Check sheet for the modelled part. Datum: model origin and axes. Units: mm. A direction names the side the tool comes from. Round coordinates to 2 decimals unless told otherwise and drop trailing zeros. Write each loop counter-clockwise with the first axis right and the second up, starting at its lowest first coordinate (ties: lowest second). Pieces come first, ordered by that corner, then holes.
Item 1: Set-up check for faces 5 (the flat face through (2, 16, 15)), 6 (the flat face through (3, 25, 7)): record each of +Z, -Z, +X, -X, +Y, -Y from which the full face is reachable in a straight line by a thin tool's end or side.
Item 2: Depth check by flat-ended pin: pin 1 (2 mm diameter, centred on x = 1, y = 120, fed in from -Z); pin 2 (12 mm diameter, centred on y = -17, z = -0.5, fed in from +X); pin 3 (5 mm diameter, centred on x = 63, z = -11.5, fed in from +Y); pin 4 (1 mm diameter, centred on y = 56.5, z = -5, fed in from -X). Enter the tip coordinate at first touch or a pass-through.
Item 3: Section check B-B, the plane y = -55. Record the cut outline in (x, z).
Item 4: Material ranges on line 1 along Z through (x, y) = (30.5, -84.3); line 2 along Y through (x, z) = (1.6, 0); line 3 along Y through (x, z) = (95, -4), recorded low to high.
Item 5: Section check A-A, the plane x = 67.5. Record the cut outline in (y, z), plus the area to 3 significant figures.
Item 6: Section check C-C, the plane x = 85. Record the cut outline in (y, z).
Item 7: Section check D-D, the plane y = 47.5. Record the cut outline in (x, z).
Item 8: Release check for a two-part mould opening along Y. For faces 1 (the cylindrical face through (1.52, 131.99, 12.15)), 2 (the cylindrical face through (1.48, 67.07, -0.65)), 3 (the flat face through (51, -85, 10)), 4 (the flat face through (0, 23, 7)) record: pulls with the +Y half, pulls with the -Y half, needs draft (parallel to the pull), parting line crosses it, or undercut.
from build123d import *

# Parameters (mm, degrees)
SKETCH_1_W          = 30
SKETCH_1_H          = 170
EXTRUDE_1_DEPTH     = 3
SKETCH_2_W          = 30
SKETCH_2_H          = 3
EXTRUDE_2_DEPTH     = 100
SKETCH_4_R          = 1.6
SKETCH_4_R_2        = 3
CUT_EXTRUDE_1_DEPTH = 104
SKETCH_5_W          = 3
SKETCH_5_H          = 30
EXTRUDE_3_DEPTH     = 50
SKETCH_6_R          = 10.5
SKETCH_6_W          = 2
SKETCH_6_H          = 2.5
CUT_EXTRUDE_2_DEPTH = 104
FILLET_1_R          = 10
SKETCH_7_R          = 1.6
SKETCH_7_W          = 60
SKETCH_7_H          = 15
CUT_EXTRUDE_3_DEPTH = 4
FILLET_2_R          = 5
SKETCH_8_R          = 5
SKETCH_8_W          = 10
SKETCH_8_H          = 60
CUT_EXTRUDE_4_DEPTH = 104


with BuildPart() as part:
    # 草图1 → 凸台-拉伸1 (new body)
    with BuildSketch(Plane(origin=(0, 0, 0), x_dir=(0, 0, -1), z_dir=(1, 0, 0))):
        Rectangle(SKETCH_1_W, SKETCH_1_H)
    extrude(amount=EXTRUDE_1_DEPTH)

    # 草图2 → 凸台-拉伸2 (add)
    with BuildSketch(Plane(origin=(3, 0, 0), x_dir=(0, 0, -1), z_dir=(1, 0, 0))):
        with Locations((0, -83.5)):
            Rectangle(SKETCH_2_W, SKETCH_2_H)
    extrude(amount=EXTRUDE_2_DEPTH)

    # 草图4 → 切除-拉伸1 (cut, through all)
    with BuildSketch(Plane.ZY):
        with Locations((-4.949747468, 74.949747468)):
            Circle(SKETCH_4_R)
        with Locations((4.949747468, 74.949747468)):
            Circle(SKETCH_4_R)
        with Locations((4.949747468, 65.050252532)):
            Circle(SKETCH_4_R)
        with Locations((-4.949747468, 65.050252532)):
            Circle(SKETCH_4_R)
        with Locations((0, 70)):
            Circle(SKETCH_4_R_2)
    extrude(amount=-CUT_EXTRUDE_1_DEPTH, mode=Mode.SUBTRACT)

    # 草图5 → 凸台-拉伸3 (add)
    with BuildSketch(Plane(origin=(0, 85, 0), x_dir=(1, 0, 0), z_dir=(0, 1, 0))):
        with Locations((1.5, 0)):
            Rectangle(SKETCH_5_W, SKETCH_5_H)
    extrude(amount=EXTRUDE_3_DEPTH)

    # 草图6 → 切除-拉伸2 (cut, through all)
    with BuildSketch(Plane.ZY):
        with Locations((0, 120)):
            Circle(SKETCH_6_R)
        with Locations((-15, 120)):
            Rectangle(SKETCH_6_W, SKETCH_6_H)
        with Locations((15, 120)):
            Rectangle(SKETCH_6_W, SKETCH_6_H)
    extrude(amount=-CUT_EXTRUDE_2_DEPTH, mode=Mode.SUBTRACT)

    # 圆角1
    fillet_1_edges = [part.edges().sort_by_distance(p)[0] for p in [
        (1.5, 135, 15),
        (1.5, 135, -15),
    ]]
    fillet(fillet_1_edges, radius=FILLET_1_R)

    # 草图7 → 切除-拉伸3 (cut, through all)
    with BuildSketch(Plane(origin=(0, -82, 0), x_dir=(1, 0, 0), z_dir=(0, 1, 0))):
        with Locations((90.5, 11.5)):
            Circle(SKETCH_7_R)
        with Locations((30.5, 11.5)):
            Circle(SKETCH_7_R)
        with Locations((90.5, -11.5)):
            Circle(SKETCH_7_R)
        with Locations((30.5, -11.5)):
            Circle(SKETCH_7_R)
        with Locations((53, 0)):
            Rectangle(SKETCH_7_W, SKETCH_7_H)
    extrude(amount=-CUT_EXTRUDE_3_DEPTH, mode=Mode.SUBTRACT)

    # 圆角2
    fillet_2_edges = [part.edges().sort_by_distance(p)[0] for p in [
        (103, -83.5, 15),
        (103, -83.5, -15),
    ]]
    fillet(fillet_2_edges, radius=FILLET_2_R)

    # 草图8 → 切除-拉伸4 (cut, through all)
    with BuildSketch(Plane.ZY):
        with Locations((0, -55)):
            Circle(SKETCH_8_R)
        Rectangle(SKETCH_8_W, SKETCH_8_H)
    extrude(amount=-CUT_EXTRUDE_4_DEPTH, mode=Mode.SUBTRACT)


solid = part.part
Values found:
1. face 5: +Z, +X, -X, +Y, -Y
1. face 6: +Z, -Z, +X, +Y
2. pin 1: stops at z = -14
2. pin 2: stops at x = 3
2. pin 3: stops at y = -82
2. pin 4: stops at x = 0
3. outline: (0, -15) - (3, -15) - (3, -5) - (0, -5) - close; (0, 5) - (3, 5) - (3, 15) - (0, 15) - close
4. line 1: z = -15 to -13.1, -9.9 to -7.5, 7.5 to 9.9, 13.1 to 15
4. line 2: y = -85 to -60, -50 to -30, 30 to 67, 73 to 109.5, 130.5 to 135
4. line 3: y = -85 to -82
5. outline: (-85, -15) - (-82, -15) - (-82, -7.5) - (-85, -7.5) - close; (-85, 7.5) - (-82, 7.5) - (-82, 15) - (-85, 15) - close
5. area: 45.0 mm2
6. outline: (-85, -15) - (-82, -15) - (-82, 15) - (-85, 15) - close
7. outline: (0, -15) - (3, -15) - (3, 15) - (0, 15) - close
8. face 1: pulls with the +Y half
8. face 2: undercut
8. face 3: pulls with the -Y half
8. face 4: needs draft
